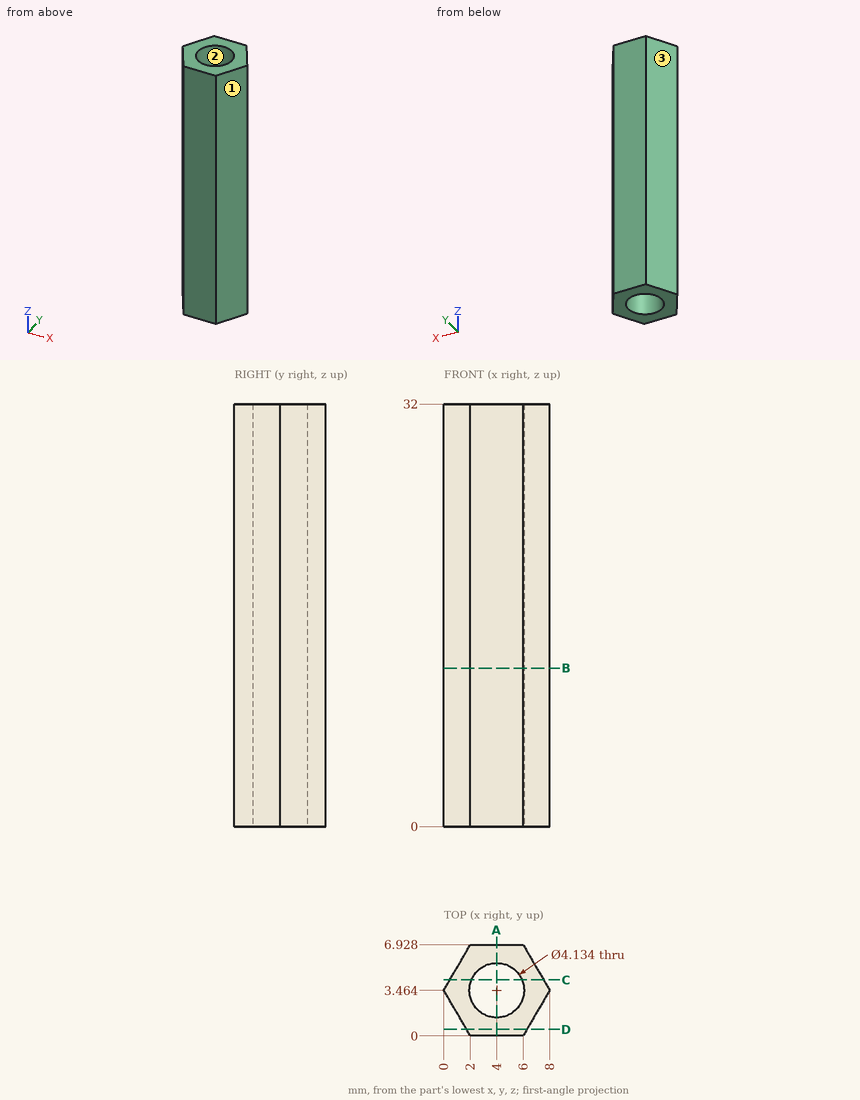
Job drawing, mm, ordinate dimensions from the low corner. One solid piece. Coordinates: 2 decimals unless noted, no trailing zeros. Write each loop counter-clockwise with the first axis right and the second up, starting at its lowest first coordinate (ties: lowest second). Pieces come first, ordered by that corner, then holes.
Item 1: Slice it at A-A (x = 4). Write the cut outline in (y, z).
Item 2: Slice it at B-B (z = 12). Write the cut outline in (x, y).
Item 3: Slice it at D-D (y = 0.5). Write the cut outline in (x, z).
Item 4: Pin check, flat tip, straight feed: pin 1 (1 mm diameter, centred on y = 4.5, z = 27, fed in from -X). Stop position of the tip, or through.
Item 5: Mould opens along Y. For the marked faces 1, 2 and 3 say: released by +Y, released by -Y, zero draft, split by the parting line, or undercut.
Item 6: Probe line 1 (X direction, y = 3.5, z = 25.5); line 2 (Y direction, x = 4.5, z = 5.5); line 3 (X direction, y = 1.75, z = 6) (1 decimal). List the from-to ranges inside material, lowest first.
Item 7: Slice it at C-C (y = 4.25). Write the cut outline in (x, z).
Results found:
1. outline: (0, 0) - (1.4, 0) - (1.4, 32) - (0, 32) - close; (5.53, 0) - (6.93, 0) - (6.93, 32) - (5.53, 32) - close
2. outline: (0, 3.46) - (2, 0) - (6, 0) - (8, 3.46) - (6, 6.93) - (2, 6.93) - close; hole circle Ø4.13 at (4, 3.46)
3. outline: (1.71, 0) - (6.29, 0) - (6.29, 32) - (1.71, 32) - close
4. pin 1: stops at x = 0.31
5. face 1: released by -Y
5. face 2: undercut
5. face 3: released by +Y
6. line 1: x = 0.02 to 1.93, 6.07 to 7.98
6. line 2: y = 0 to 1.46, 5.47 to 6.93
6. line 3: x = 1 to 2.8, 5.2 to 7
7. outline: (0.45, 0) - (2.09, 0) - (2.09, 32) - (0.45, 32) - close; (5.91, 0) - (7.55, 0) - (7.55, 32) - (5.91, 32) - close
